For this review, take the finished solid that the model builds, in its own axes (mm). Coordinates: 2 decimals unless noted, no trailing zeros. Loops run counter-clockwise (first coordinate to the right, second up) from the corner with the lowest first, then second, coordinate; pieces in that order, holes last. Notation, with made-up numbers: (10.5, 41) -> (21.5, 41) arc R26 ccw to (21.5, 63) -> close; hole circle Ø2 at (-36, -22.5). An arc over 180 degrees is marked (long way). One line per item, written item: value.
Autodesk Inventor part; units mm, degrees
ref_plane "YZ Plane" through (0, 0, 0) normal (1, 0, 0) x (0, 1, 0)
ref_plane "XZ Plane" through (0, 0, 0) normal (0, 1, 0) x (-1, 0, 0)
ref_plane "XY Plane" through (0, 0, 0) normal (0, 0, 1) x (1, 0, 0)
sketch "Sketch1" plane through (0, 0, 0) normal (0, 0, 1) x (1, 0, 0)
  line L0 (1.3568, 2.35) -> (2.7135, 0)
  line L1 (2.7135, 0) -> (1.3568, -2.35)
  line L2 (1.3568, -2.35) -> (-1.3568, -2.35)
  line L3 (-1.3568, -2.35) -> (-2.7135, 0)
  line L4 (-2.7135, 0) -> (-1.3568, 2.35)
  line L5 (-1.3568, 2.35) -> (1.3568, 2.35)
  circle A0 centre (0, 0) radius 1.5
  point P0 (0, 2.35)
  dimension "d0" = 4.7
  dimension "d1" = 3
extrude "Extrusion1" add sketch "Sketch1" along normal mid plane 12
properties part number "spacerHex" material "Brass, Soft Yellow, Welded"
1. Take a section at C-C, the plane y = 0.35. Give the boundary of the cut face in (x, z).
Return value:
outline: (-2.51, -6) -> (-1.46, -6) -> (-1.46, 6) -> (-2.51, 6) -> close; (1.46, -6) -> (2.51, -6) -> (2.51, 6) -> (1.46, 6) -> close
2. Take a section at B-B, the plane x = -1.2. Give the boundary of the cut face in (y, z), and give its area (3 significant figures).
Return value:
outline: (-2.35, -6) -> (-0.9, -6) -> (-0.9, 6) -> (-2.35, 6) -> close; (0.9, -6) -> (2.35, -6) -> (2.35, 6) -> (0.9, 6) -> close
area: 34.8 mm2
3. The part is to be moulded in two halves that separate along Y. For faces 1 (the flat face through (-2.026, -1.191, -0.084)), 2 (the cylindrical face through (-1.5, -0.07, -0.08)), 3 (the flat face through (-2.045, 1.159, -0.084)), say which applies: pulls with the +Y half, pulls with the -Y half, needs draft (parallel to the pull), parting line crosses it, or undercut.
Return value:
face 1: pulls with the -Y half
face 2: undercut
face 3: pulls with the +Y half
4. Take a section at D-D, the plane x = 1.75. Give the boundary of the cut face in (y, z).
Return value:
outline: (-1.67, -6) -> (1.67, -6) -> (1.67, 6) -> (-1.67, 6) -> close
5. To check wall thickness, follow probe 1 along Y at (x, z) = (0, 1.75); probe 2 along Y at (x, z) = (-1.2, -0.5); probe 3 along X at (y, z) = (-0.5, 5). State the ranges of each line that lie inside material, in increasing order. Write a range as from..to.
Return value:
probe 1: y = -2.35..-1.5, 1.5..2.35
probe 2: y = -2.35..-0.9, 0.9..2.35
probe 3: x = -2.42..-1.41, 1.41..2.42
6. Take a section at A-A, the plane z = -0.25. Give the boundary of the cut face in (x, y), and give its area (3 significant figures).
Return value:
outline: (-2.71, 0) -> (-1.36, -2.35) -> (1.36, -2.35) -> (2.71, 0) -> (1.36, 2.35) -> (-1.36, 2.35) -> close; hole circle Ø3 at (0, 0)
area: 12.1 mm2
